```python
from build123d import *

# Parameters (mm, degrees)
EXTRUDE_1_DEPTH     = 10
SKETCH_2_R          = 5
CUT_EXTRUDE_1_DEPTH = 3.5
CUT_EXTRUDE_START   = -3.5
SKETCH_3_R          = 5
CUT_EXTRUDE_2_DEPTH = 3.5
SKETCH_4_R          = 1.6
CUT_EXTRUDE_3_DEPTH = 10


with BuildPart() as part:
    # 草图1 → 凸台-拉伸1 (new body)
    with BuildSketch(Plane(origin=(0, 0, 0), x_dir=(1, 0, 0), z_dir=(0, 1, 0))):
        with BuildLine():
            Line((0, 0), (0, 25))
            ThreePointArc((0, 25), (10, 35), (20, 25))
            Line((20, 25), (20, 0))
            Line((20, 0), (0, 0))
        make_face()
    extrude(amount=EXTRUDE_1_DEPTH)

    # 草图2 → 切除-拉伸1 (cut)
    with BuildSketch(Plane(origin=(0, 0, 0), x_dir=(1, 0, 0), z_dir=(0, 1, 0))):
        with Locations(Location((10, 25, 0), (0, 0, 270))):
            Circle(SKETCH_2_R)
    extrude(amount=CUT_EXTRUDE_1_DEPTH, mode=Mode.SUBTRACT)

    # 草图3 → 切除-拉伸2 (cut)
    with BuildSketch(Plane(origin=(0, 10, 0), x_dir=(1, 0, 0), z_dir=(0, 1, 0)).offset(CUT_EXTRUDE_START)):
        with Locations(Location((10, 25, 0), (0, 0, 270))):
            Circle(SKETCH_3_R)
    extrude(amount=CUT_EXTRUDE_2_DEPTH, mode=Mode.SUBTRACT)

    # 草图4 → 切除-拉伸3 (cut)
    with BuildSketch(Plane.XY):
        with Locations((6, 5)):
            Circle(SKETCH_4_R)
        with Locations((14, 5)):
            Circle(SKETCH_4_R)
    extrude(amount=-CUT_EXTRUDE_3_DEPTH, mode=Mode.SUBTRACT)


solid = part.part
```
Geometry check sheet. Reference: the model listing, model coordinates, mm. A direction names the side the tool comes from. Coordinates: 2 decimals unless noted, no trailing zeros. Order: outer loops, then holes, each group sorted by start corner. A loop starts at its lowest first (then second) coordinate and runs counter-clockwise, first axis right, second up.
Item 1: Scan lines: line 1 along X through (y, z) = (1.55, -25); line 2 along Y through (x, z) = (6, -7.5); line 3 along Y through (x, z) = (13.5, -5). Record each from-to range of solid material in increasing order.
Item 2: Section check D-D (z = -31.5). Enter the section's corners in (x, y).
Item 3: Section check C-C (y = 5). Enter the section's corners in (x, z).
Item 4: Tool access check on faces 4 (the cylindrical face through (6.74, 3.58, -4.93)), 5 (the flat face through (10, 10, -14)), 6 (the flat face through (10, 3.5, -25)), 7 (the cylindrical face through (10, 8, -30)). Record the directions out of +Z, -Z, +X, -X, +Y, -Y that give a thin tool (end or side, any length) a straight path to the whole face; none if there is none.
Item 5: Section check A-A (y = 8.25). Enter the section's corners in (x, z).
Item 6: Section check B-B (x = 10). Enter the section's corners in (y, z).
Item 7: Mould release check, pull along Y, two halves, no side actions. Record for faces 1 (the flat face through (10, 6.5, -25)), 2 (the flat face through (14, 5, -10)), 3 (the cylindrical face through (10, 2, -30)): released by +Y, released by -Y, zero draft, split by the parting line, or undercut.
Item 8: Depth check by flat-ended pin: pin 1 (1 mm diameter, centred on x = 17.5, y = 9, fed in from -Z); pin 2 (9 mm diameter, centred on x = 10, z = -25, fed in from +Y); pin 3 (5 mm diameter, centred on x = 5.5, y = 7.5, fed in from -Z). Enter the tip coordinate at first touch or a pass-through.
Check sheet entries:
1. line 1: x = 0 to 5, 15 to 20
1. line 2: y = 0 to 3.4, 6.6 to 10
1. line 3: y = 0 to 3.48, 6.52 to 10
2. outline: (2.4, 0) - (17.6, 0) - (17.6, 10) - (2.4, 10) - close
3. outline: (0, -25) arc R10 ccw to (20, -25) - (20, 0) - (15.6, 0) - (15.6, -10) - (12.4, -10) - (12.4, 0) - (7.6, 0) - (7.6, -10) - (4.4, -10) - (4.4, 0) - (0, 0) - close
4. face 4: +Z
4. face 5: +Z, -Z, +X, -X, +Y
4. face 6: -Y
4. face 7: +Y
5. outline: (0, -25) arc R10 ccw to (20, -25) - (20, 0) - (0, 0) - close; hole circle Ø10 at (10, -25)
6. outline: (0, -35) - (10, -35) - (10, -30) - (6.5, -30) - (6.5, -20) - (10, -20) - (10, 0) - (0, 0) - (0, -20) - (3.5, -20) - (3.5, -30) - (0, -30) - close
7. face 1: released by +Y
7. face 2: undercut
7. face 3: zero draft
8. pin 1: stops at z = -32.14
8. pin 2: stops at y = 6.5
8. pin 3: stops at z = -34.8
